Could you check a few things on this model? Use its own coordinates, in mm. A direction names the side the tool comes from. Round coordinates to 2 decimals unless told otherwise and drop trailing zeros. Write each loop counter-clockwise with the first axis right and the second up, starting at its lowest first coordinate (ties: lowest second). Pieces come first, ordered by that corner, then holes. Notation, with made-up numbers: (49, 39) - (78, 39) arc R24 cw to (78, 77) - close; hole circle Ø5 at (36.5, -20.5). An arc over 180 degrees is marked (long way). Write each question's results on one line, items separated by ' | '. Start each with the question number.
(1) Imagine slicing it at B-B on y = 99. Write out the boundary of the cut face in (x, z).
(2) Imagine slicing it at C-C on x = -150. Write out the boundary of the cut face in (y, z).
(3) Please list where these lines run through material, in increasing order: line 1 (X direction, y = -51.5, z = 0.5); line 2 (Z direction, x = -81, y = -4.5); line 3 (Y direction, x = 1, z = 49). Write a range as [from, to].
(4) On a 3-axis mill with a long thin cutter (end or side, diameter ignored), from which of +Z, -Z, +X, -X, +Y, -Y can I reach the whole of each face in a straight line? I mean faces 1 (the flat face through (-25, -50, 5)), 2 (the flat face through (10, -62, 30)), 3 (the flat face through (25, -50, 5)), 4 (the flat face through (0, 60, 45)). Say none if no direction works.
(5) Imagine slicing it at D-D on z = -70. Write out the boundary of the cut face in (x, y), then the cut area to 3 significant figures.
(6) For P1, Ø11, axis at x = -32.5, z = 6, coming from the +Y side; P2, Ø16, axis at x = 40, y = 40, coming from the +Z side; P3, Ø6, axis at x = -2.5, z = 46, coming from the -Y side, each with a flat end and sliding along its axis, tell me the tip position at first contact or that it passes through.
(7) Imagine slicing it at A-A on z = 54. Write out the boundary of the cut face in (x, y).
(8) Thinking about a two-plate mould opening in Z: for faces 5 (the flat face through (0, 0, -100)), 6 (the cylindrical face through (1.302, 75.103, 69.915)), 7 (the flat face through (-134, 0, 4)), 8 (the flat face through (-10, -62, 30)), which applies, +Z half, -Z half, draft (parallel to the pull), parting line (faces both ways), or undercut?
```python
from build123d import *

# Parameters (mm, degrees)
BOSS_EXTRUDE1_DEPTH  = 10
CUT_EXTRUDE1_DEPTH   = 10
SKETCH6_W            = 20
SKETCH6_H            = 10
BOSS_EXTRUDE5_DEPTH  = 10
SKETCH7_W            = 20
SKETCH7_H            = 10
BOSS_EXTRUDE6_DEPTH  = 60
FILLET7_R            = 20
FILLET8_R            = 10
BOSS_EXTRUDE7_DEPTH  = 10
CUT_EXTRUDE7_DEPTH   = 18
FILLET7_OF_MIRROR2_R = 20
FILLET8_OF_MIRROR2_R = 10
SKETCH19_R           = 5
CUT_EXTRUDE9_DEPTH   = 30
SKETCH29_R           = 10
BOSS_EXTRUDE16_DEPTH = 15
SKETCH31_R           = 10
BOSS_EXTRUDE17_DEPTH = 15
BOSS_EXTRUDE21_DEPTH = 10
FILLET9_R            = 10
FILLET10_R           = 10
SKETCH35_R           = 10
CUT_EXTRUDE11_DEPTH  = 30
SKETCH16_R           = 25
BOSS_EXTRUDE22_DEPTH = 100


with BuildPart() as part:
    # Sketch2 → Boss-Extrude1 (new body)
    with BuildSketch(Plane.XY):
        with BuildLine():
            Line((-40, 50), (40, 50))
            ThreePointArc((40, 50), (47.071067812, 47.071067812), (50, 40))
            Line((50, 40), (50, -40))
            ThreePointArc((50, -40), (47.071067812, -47.071067812), (40, -50))
            Line((40, -50), (-40, -50))
            ThreePointArc((-40, -50), (-47.071067812, -47.071067812), (-50, -40))
            Line((-50, -40), (-50, 40))
            ThreePointArc((-50, 40), (-47.071067812, 47.071067812), (-40, 50))
        make_face()
    boss_extrude1 = extrude(amount=BOSS_EXTRUDE1_DEPTH)

    # Sketch3 → Cut-Extrude1 (cut)
    with BuildSketch(Plane.XY.offset(10)):
        with BuildLine():
            Line((-50, 40), (-50, -40))
            ThreePointArc((-50, -40), (-39.282032303, 0), (-50, 40))
        make_face()
        with BuildLine():
            Line((50, 40), (50, -40))
            ThreePointArc((50, -40), (39.282032303, 0), (50, 40))
        make_face()
    cut_extrude1 = extrude(amount=-CUT_EXTRUDE1_DEPTH, mode=Mode.SUBTRACT)

    # Sketch6 → Boss-Extrude5 (add)
    with BuildSketch(Plane.XZ.offset(50)):
        with Locations((0, 5)):
            Rectangle(SKETCH6_W, SKETCH6_H)
    boss_extrude5 = extrude(amount=BOSS_EXTRUDE5_DEPTH)

    # Sketch7 → Boss-Extrude6 (add)
    with BuildSketch(Plane.XY):
        with Locations((0, -65)):
            Rectangle(SKETCH7_W, SKETCH7_H)
    boss_extrude6 = extrude(amount=BOSS_EXTRUDE6_DEPTH)

    # Fillet7
    fillet7_edges = [part.edges().sort_by_distance(p)[0] for p in [
        (0, -70, 0),
    ]]
    fillet(fillet7_edges, radius=FILLET7_R)

    # Fillet8
    fillet8_edges = [part.edges().sort_by_distance(p)[0] for p in [
        (0, -60, 10),
    ]]
    fillet(fillet8_edges, radius=FILLET8_R)

    # Sketch8 → Boss-Extrude7 (add)
    with BuildSketch(Plane(origin=(0, -60, 0), x_dir=(1, 0, 0), z_dir=(0, 1, 0))):
        with BuildLine():
            Line((10, -60), (-10, -60))
            ThreePointArc((-10, -60), (0, -70), (10, -60))
        make_face()
    boss_extrude7 = extrude(amount=-BOSS_EXTRUDE7_DEPTH)

    # Sketch14 → Cut-Extrude7 (cut)
    with BuildSketch(Plane.XY.offset(10)):
        with BuildLine():
            Line((-39.282032303, 0), (39.282032303, 0))
            add(Edge.make_bspline(
                [(50, 40), (39.359472874, 21.350658255), (39.282032303, 0)],
                knots=[0, 0, 0, 1, 1, 1], degree=2))
            add(Edge.make_bspline(
                [(40, 50), (49.142135624, 49.142135624), (50, 40)],
                knots=[0, 0, 0, 1, 1, 1], degree=2))
            Line((40, 50), (-40, 50))
            add(Edge.make_bspline(
                [(-50, 40), (-49.142135624, 49.142135624), (-40, 50)],
                knots=[0, 0, 0, 1, 1, 1], degree=2))
            add(Edge.make_bspline(
                [(-39.282032303, 0), (-39.359472874, 21.350658255), (-50, 40)],
                knots=[0, 0, 0, 1, 1, 1], degree=2))
        make_face()
    extrude(amount=-CUT_EXTRUDE7_DEPTH, mode=Mode.SUBTRACT)


with BuildPart() as cut_extrude7_kept_piece:
    # of the separate pieces the step leaves, the one the design keeps (cut_extrude7_pieces_kept)
    add(part.part.solids().sort_by_distance((-10, -60, 20))[0])

    # Mirror2: Boss-Extrude1, Cut-Extrude1, Boss-Extrude5, Boss-Extrude6, Boss-Extrude7 across plane
    add(boss_extrude1.mirror(Plane(origin=(-39.282032303, 0, -8), x_dir=(0, 0, 1), z_dir=(0, -1, 0))))
    add(cut_extrude1.mirror(Plane(origin=(-39.282032303, 0, -8), x_dir=(0, 0, 1), z_dir=(0, -1, 0))), mode=Mode.SUBTRACT)
    add(boss_extrude5.mirror(Plane(origin=(-39.282032303, 0, -8), x_dir=(0, 0, 1), z_dir=(0, -1, 0))))
    add(boss_extrude6.mirror(Plane(origin=(-39.282032303, 0, -8), x_dir=(0, 0, 1), z_dir=(0, -1, 0))))
    add(boss_extrude7.mirror(Plane(origin=(-39.282032303, 0, -8), x_dir=(0, 0, 1), z_dir=(0, -1, 0))))

    # Fillet7 of Mirror2
    fillet7_of_mirror2_edges = [cut_extrude7_kept_piece.edges().sort_by_distance(p)[0] for p in [
        (0, 70, 0),
    ]]
    fillet(fillet7_of_mirror2_edges, radius=FILLET7_OF_MIRROR2_R)

    # Fillet8 of Mirror2
    fillet8_of_mirror2_edges = [cut_extrude7_kept_piece.edges().sort_by_distance(p)[0] for p in [
        (0, 60, 10),
    ]]
    fillet(fillet8_of_mirror2_edges, radius=FILLET8_OF_MIRROR2_R)

    # Sketch19 → Cut-Extrude9 (cut)
    with BuildSketch(Plane.XY.offset(10)):
        with Locations((-40, 40)):
            Circle(SKETCH19_R)
        with Locations((40, 40)):
            Circle(SKETCH19_R)
        with Locations((-40, -40)):
            Circle(SKETCH19_R)
        with Locations((40, -40)):
            Circle(SKETCH19_R)
    extrude(amount=-CUT_EXTRUDE9_DEPTH, mode=Mode.SUBTRACT)

    # Sketch29 → Boss-Extrude16 (add)
    with BuildSketch(Plane(origin=(0, 70, 0), x_dir=(1, 0, 0), z_dir=(0, 1, 0))):
        with Locations(Location((0, -60, 0), (0, 0, 180))):
            Circle(SKETCH29_R)
    extrude(amount=BOSS_EXTRUDE16_DEPTH)

    # Sketch30 → Revolve2 (revolve)
    with BuildSketch(Plane(origin=(0, 0, 0), x_dir=(0, 0, -1), z_dir=(1, 0, 0))):
        with BuildLine():
            Line((-60, 118.027756377), (-60, 85))
            Line((-60, 85), (-50, 85))
            ThreePointArc((-50, 85), (-42.745778116, 105.224158035), (-60, 118.027756377))
        make_face()
    revolve(axis=Axis((0, 85, 60), (0, 1, 0)))

    # Sketch31 → Boss-Extrude17 (add)
    with BuildSketch(Plane.XZ.offset(70)):
        with Locations(Location((0, 60, 0), (0, 0, 180))):
            Circle(SKETCH31_R)
    extrude(amount=BOSS_EXTRUDE17_DEPTH)

    # Sketch32 → Revolve3 (revolve)
    with BuildSketch(Plane(origin=(0, 0, 0), x_dir=(0, 0, -1), z_dir=(1, 0, 0))):
        with BuildLine():
            Line((-60, -118.027756377), (-60, -85))
            Line((-60, -85), (-70, -85))
            ThreePointArc((-70, -85), (-77.254221884, -105.224158035), (-60, -118.027756377))
        make_face()
    revolve(axis=Axis((0, -85, 60), (0, -1, 0)))

    # Sketch33 → Boss-Extrude21 (add)
    with BuildSketch(Plane.XY.offset(10)):
        with BuildLine():
            Line((-134, 10), (-39.909492971, 10))
            ThreePointArc((-39.909492971, 10), (-39.282032303, 0), (-39.909492971, -10))
            Line((-39.909492971, -10), (-134, -10))
            Line((-134, -10), (-134, 10))
        make_face()
    extrude(amount=-BOSS_EXTRUDE21_DEPTH)

    # Sketch34 → Revolve5 (revolve)
    with BuildSketch(Plane.XY):
        with BuildLine():
            Line((-178, 0), (-168.867962264, 0))
            ThreePointArc((-168.867962264, 0), (-155.201567253, 18.136805069), (-134, 10))
            Line((-134, 10), (-123.846606339, 10))
            ThreePointArc((-123.846606339, 10), (-155.08453427, 27.534478591), (-178, 0))
        make_face()
    revolve(axis=Axis((-134, 0, 0), (-1, 0, 0)))

    # Fillet9
    # the kernel refuses this fillet: 10 mm, written as the material it adds along each edge
    with BuildSketch(Plane(origin=(-150, 10, 0), x_dir=(1, 0, 0), z_dir=(0, 0, -1))) as fillet9_piece_1_section:
        with BuildLine():
            CenterArc((32.310988843, -10), FILLET9_R, 90, 58.243136141)
            ThreePointArc((23.808097042, -4.736842105), (25.09276901, -2.423886002), (26.153393661, 0))
            Line((26.153393661, 0), (32.310988843, 0))
        make_face()
    fillet9_piece_1 = revolve(axis=Axis((-150, 10, 0), (0, -1, 0)), revolution_arc=56.205276657, mode=Mode.PRIVATE)
    fillet9_piece_1 = split(fillet9_piece_1, bisect_by=Plane(origin=(-123.595029593, 11.027181376, 10), z_dir=(0, 0, -1)), keep=Keep.TOP, mode=Mode.PRIVATE)
    add(fillet9_piece_1)

    # Fillet10
    # the kernel refuses this fillet: 10 mm, written as the material it adds along each edge
    with BuildSketch(Plane(origin=(-150, -10, 0), x_dir=(0.5562190835944724, 0, 0.8310356978164808), z_dir=(-0.8310356978164808, 0, 0.5562190835944724))) as fillet10_piece_1_section:
        with BuildLine():
            CenterArc((32.310988843, -10), FILLET10_R, 90, 58.243136141)
            ThreePointArc((23.808097042, -4.736842105), (25.09276901, -2.423886002), (26.153393661, 0))
            Line((26.153393661, 0), (32.310988843, 0))
        make_face()
    fillet10_piece_1 = revolve(axis=Axis((-150, -10, 0), (0, 1, 0)), revolution_arc=56.205276657, mode=Mode.PRIVATE)
    fillet10_piece_1 = split(fillet10_piece_1, bisect_by=Plane(origin=(-123.595029593, -11.027181376, 10), z_dir=(0, 0, -1)), keep=Keep.TOP, mode=Mode.PRIVATE)
    add(fillet10_piece_1)

    # Sketch35 → Cut-Extrude11 (cut)
    with BuildSketch(Plane.XY):
        with Locations(Location((-150, 0, 0), (0, 0, 180))):
            Circle(SKETCH35_R)
    extrude(amount=CUT_EXTRUDE11_DEPTH, mode=Mode.SUBTRACT)

    # Sketch16 → Boss-Extrude22 (add)
    with BuildSketch(Plane(origin=(0, 0, 0), x_dir=(-1, 0, 0), z_dir=(0, 0, -1))):
        with Locations(Location((0, 0, 0), (0, 0, 180))):
            Circle(SKETCH16_R)
    extrude(amount=BOSS_EXTRUDE22_DEPTH)


solid = cut_extrude7_kept_piece.part
```
Response:
1) outline: circle Ø36 at (0, 60)
2) outline: (-10, 16) - (-10, 26.15) arc R28 ccw (long way) to (10, 26.15) - (10, 16) arc R18.87 cw (long way) to start
3) line 1: [-10, 10] | line 2: [0, 10] | line 3: [-114.25, -85.75], [-70, -60], [60, 70], [85.75, 114.25]
4) face 1: +Z, -Z, -X, -Y | face 2: +Z, -Z, +X | face 3: +Z, -Z, +X, -Y | face 4: +Z, +X, -X
5) outline: circle Ø50 at (0, 0) | area: 1,960 mm²
6) P1: y = 50 | P2: z = 10 | P3: y = -114.11
7) outline: (-10, -70) - (-8, -70) - (-8, -85) arc R17 ccw (long way) to (8, -85) - (8, -70) - (10, -70) - (10, -60) - (-10, -60) - close; (-10, 60) - (10, 60) - (10, 70) - (8, 70) - (8, 85) arc R17 ccw (long way) to (-8, 85) - (-8, 70) - (-10, 70) - close
8) face 5: -Z half | face 6: parting line | face 7: undercut | face 8: draft
